Verification items for this drawing (mm, ordinates from the low corner). Round coordinates to 2 decimals unless told otherwise and drop trailing zeros. Order: outer loops, then holes, each group sorted by start corner. A loop starts at its lowest first (then second) coordinate and runs counter-clockwise, first axis right, second up. Notation, with made-up numbers: (9.5, 51) -> (61.5, 51) arc R14 ccw to (61.5, 59) -> close; hole circle Ø8 at (85.5, -7). An arc over 180 degrees is marked (long way). Answer in a Markdown table with one row per item. Add a question column.
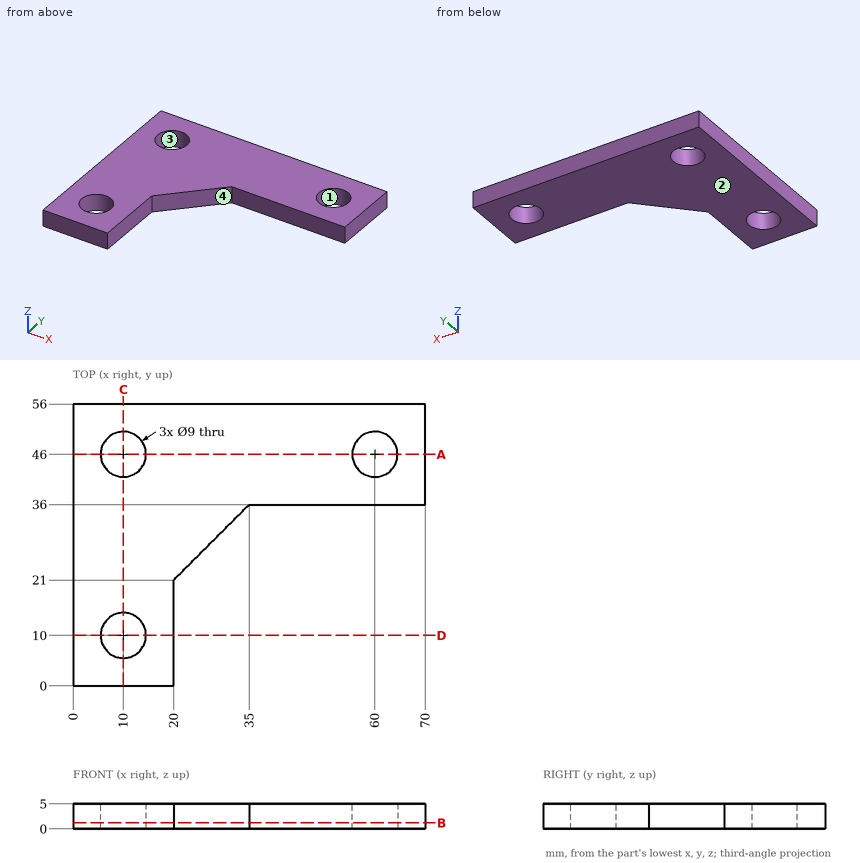
1) Cross-section at C-C, the plane x = 10. Record the boundary of the cut face in (y, z), and give its area (3 significant figures).
2) Depth check by flat-ended pin: P1, Ø2.5, axis at x = 52.5, z = 2, coming from the -Y side; P2, Ø1, axis at y = 21.5, z = 1.5, coming from the +X side; P3, Ø1.5, axis at y = 23, z = 1.5, coming from the +X side; P4, Ø8, axis at x = 10, y = 10, coming from the -Z side. Enter the tip coordinate at first touch or a pass-through.
3) Draft check along Y on the marked faces 1, 2, 3 and 4. Enter one of: +Y half, -Y half, draft (parallel to the pull), parting line (faces both ways), or undercut.
4) Cross-section at B-B, the plane z = 1.2. Record the boundary of the cut face in (x, y), and give its area (3 significant figures).
5) Cross-section at D-D, the plane y = 10. Record the boundary of the cut face in (x, z), and give its area (3 significant figures).
6) Cross-section at A-A, the plane y = 46. Record the boundary of the cut face in (x, z), and give its area (3 significant figures).
7) Thickness scan on L1, parallel to Y at x = 10, z = 2; L2, parallel to Y at x = 40, z = 0.9; L3, parallel to X at y = 16, z = 2.6. Record the ranges inside material, lowest first. Write a range as [from, to].
Results below:
| question | item | result |
|---|---|---|
| 1 | outline | (0, 0) -> (5.5, 0) -> (5.5, 5) -> (0, 5) -> close; (14.5, 0) -> (41.5, 0) -> (41.5, 5) -> (14.5, 5) -> close; (50.5, 0) -> (56, 0) -> (56, 5) -> (50.5, 5) -> close |
| 1 | area | 190 mm² |
| 2 | P1 | y = 36 |
| 2 | P2 | x = 21 |
| 2 | P3 | x = 22.75 |
| 2 | P4 | through |
| 3 | face 1 | undercut |
| 3 | face 2 | draft |
| 3 | face 3 | undercut |
| 3 | face 4 | -Y half |
| 4 | outline | (0, 0) -> (20, 0) -> (20, 21) -> (35, 36) -> (70, 36) -> (70, 56) -> (0, 56) -> close; hole circle Ø9 at (10, 10); hole circle Ø9 at (10, 46); hole circle Ø9 at (60, 46) |
| 4 | area | 2,040 mm² |
| 5 | outline | (0, 0) -> (5.5, 0) -> (5.5, 5) -> (0, 5) -> close; (14.5, 0) -> (20, 0) -> (20, 5) -> (14.5, 5) -> close |
| 5 | area | 55.0 mm² |
| 6 | outline | (0, 0) -> (5.5, 0) -> (5.5, 5) -> (0, 5) -> close; (14.5, 0) -> (55.5, 0) -> (55.5, 5) -> (14.5, 5) -> close; (64.5, 0) -> (70, 0) -> (70, 5) -> (64.5, 5) -> close |
| 6 | area | 260 mm² |
| 7 | L1 | [0, 5.5], [14.5, 41.5], [50.5, 56] |
| 7 | L2 | [36, 56] |
| 7 | L3 | [0, 20] |
